Geometry: final body of the model. Coordinates: model frame, mm. A direction names the side the tool comes from. Round coordinates to 2 decimals unless told otherwise and drop trailing zeros. Loops run counter-clockwise (first coordinate to the right, second up) from the corner with the lowest first, then second, coordinate; pieces in that order, holes last. Notation, with made-up numbers: M 76,63.25 L 119,63.25 A18 cw 119,93.25 Z; hole C 67,16.25 d11. An arc over 180 degrees is marked long. Write each question's results on one line, items separated by ' | '.
```python
from build123d import *

# Parameters (mm, degrees)
F3_R     = 1.27
F4_DEPTH = 10.16
F6_R     = 15.24
F7_DEPTH = 2.54
F8_R     = 9.525
F8_R_2   = 2.6694227638
F9_DEPTH = 25.4


with BuildPart() as f1:
    # F0 (on Front) → F1 (revolve)
    with BuildSketch(Plane.XZ):
        with BuildLine():
            Line((0, 33.3398456074), (0, 38.1))
            ThreePointArc((0, 38.1), (-5.3715700607, 37.719441076), (-10.6358330914, 36.585366671))
            ThreePointArc((-10.6358330914, 36.585366671), (-5.5599989326, 34.1692827218), (0, 33.3398456074))
        make_face()
        with BuildLine():
            ThreePointArc((-10.6358330914, 36.585366671), (-5.3715700607, 37.719441076), (0, 38.1))
            Line((0, 38.1), (0, 67.6917069877))
            ThreePointArc((0, 67.6917069877), (-3.5141843979, 68.3636773923), (-6.5325309142, 70.2847761705))
            ThreePointArc((-6.5325309142, 70.2847761705), (-18.9103339688, 54.6924027056), (-10.6358330914, 36.585366671))
        make_face()
        with BuildLine():
            ThreePointArc((0, 33.3398456074), (-5.5599989326, 34.1692827218), (-10.6358330914, 36.585366671))
            ThreePointArc((-10.6358330914, 36.585366671), (-37.719441076, -5.3715700607), (0, -38.1))
            Line((0, -38.1), (0, 33.3398456074))
        make_face()
        with BuildLine():
            ThreePointArc((-6.5325309142, 70.2847761705), (-3.5141843979, 68.3636773923), (0, 67.6917069877))
            Line((0, 67.6917069877), (0, 71.4398456074))
            ThreePointArc((0, 71.4398456074), (-3.3169317731, 71.1488558055), (-6.5325309142, 70.2847761705))
        make_face()
        with BuildLine():
            ThreePointArc((0, 86.7417069877), (-8.8530295954, 80.7308913857), (-6.5325309142, 70.2847761705))
            ThreePointArc((-6.5325309142, 70.2847761705), (-3.3169317731, 71.1488558055), (0, 71.4398456074))
            Line((0, 71.4398456074), (0, 86.7417069877))
        make_face()
    revolve(axis=Axis((0, 0, 28.575), (0, 0, -1)))

    # F3 (on offset) → F4 (join)
    with BuildSketch(Plane.YZ):
        with BuildLine():
            ThreePointArc((1.27, 73.7371481955), (0.8980256121, 74.6351738076), (0, 75.0071481955))
            Line((0, 75.0071481955), (0, 72.4671481955))
            ThreePointArc((0, 72.4671481955), (0.8980256121, 72.8391225834), (1.27, 73.7371481955))
        make_face()
        with BuildLine():
            Line((0, 72.4671481955), (0, 75.0071481955))
            ThreePointArc((0, 75.0071481955), (-1.27, 73.7371481955), (0, 72.4671481955))
        make_face()
        with BuildLine():
            ThreePointArc((1.27, 78.1989917159), (0.8980256121, 79.097017328), (0, 79.4689917159))
            Line((0, 79.4689917159), (0, 76.9289917159))
            ThreePointArc((0, 76.9289917159), (0.8980256121, 77.3009661038), (1.27, 78.1989917159))
        make_face()
        with BuildLine():
            Line((0, 76.9289917159), (0, 79.4689917159))
            ThreePointArc((0, 79.4689917159), (-1.27, 78.1989917159), (0, 76.9289917159))
        make_face()
        with BuildLine():
            ThreePointArc((-5.3214693207, 82.12595433), (-3.4164693207, 80.22095433), (-1.5114693207, 82.12595433))
            Line((-1.5114693207, 82.12595433), (-5.3214693207, 82.12595433))
        make_face()
        with BuildLine():
            Line((-5.3214693207, 82.12595433), (-1.5114693207, 82.12595433))
            ThreePointArc((-1.5114693207, 82.12595433), (-3.4164693207, 84.03095433), (-5.3214693207, 82.12595433))
        make_face()
        with BuildLine():
            ThreePointArc((5.4735306793, 82.12595433), (3.5685306793, 84.03095433), (1.6635306793, 82.12595433))
            Line((1.6635306793, 82.12595433), (5.4735306793, 82.12595433))
        make_face()
        with BuildLine():
            Line((5.4735306793, 82.12595433), (1.6635306793, 82.12595433))
            ThreePointArc((1.6635306793, 82.12595433), (3.5685306793, 80.22095433), (5.4735306793, 82.12595433))
        make_face()
        with Locations((-7.385127712, 77.2191482013)):
            Circle(F3_R)
        with Locations((-4.0002781898, 74.8141407967)):
            Circle(F3_R)
        with Locations((7.0602684917, 77.3848402455)):
            Circle(F3_R)
        with Locations((3.981257522, 74.8031953548)):
            Circle(F3_R)
    extrude(amount=F4_DEPTH)

    # F6 (on offset) → F7 (join)
    with BuildSketch(Plane.XY.offset(83.82)):
        Circle(F6_R)
    extrude(amount=F7_DEPTH)

    # F8 (on face) → F9 (join)
    with BuildSketch(Plane.XY.offset(86.36)):
        Circle(F8_R)
        Circle(F8_R_2, mode=Mode.SUBTRACT)
    extrude(amount=F9_DEPTH)


solid = f1.part
```
1. Section B-B (y = -24). Output: boundary loops of the cut face in (x, z), then the cut area to 3 significant figures.
Answer key:
outline: C 0,0 d59.18 | area: 2,750 mm²
2. Pin query (flat end, axial travel): P1, Ø1.5, axis at x = 17.5, z = -13.5, coming from the +Y side; P2, Ø1.8, axis at y = -4, z = 82, coming from the +X side; P3, Ø3, axis at y = 3.5, z = 82.5, coming from the +X side. Return the tip coordinate at first contact, or that it passes through.
Answer key:
P1: stops at y = 31.55 | P2: stops at x = 10.16 | P3: stops at x = 14.98
3. Draft query along Y for faces 1 (the face through (10.16, -3, 82)), 2 (the face through (8.252, -5.265, 82.587)), 3 (the face through (-3.3, -14.88, 85.07)). Return one class per face: pulls with the +Y half, pulls with the -Y half, needs draft (parallel to the pull), parting line crosses it, or undercut.
Answer key:
face 1: needs draft | face 2: undercut | face 3: parting line crosses it
4. Section C-C (z = 2). Output: boundary loops of the cut face in (x, y).
Answer key:
outline: C 0,0 d76.09
5. Ray query, probe 1 along Y at (x, z) = (0, 92.5) (3 decimals); probe 2 along Y at (x, z) = (-1, 104); probe 3 along Z at (x, y) = (-22.5, -25). Return the intervals inside material, ascending.
Answer key:
probe 1: y = -9.525 to -2.669, 2.669 to 9.525 | probe 2: y = -9.47 to -2.48, 2.48 to 9.47 | probe 3: z = -17.9 to 17.9
6. Access query for faces 4 (the face through (-4, -7, 83.82)), 5 (the face through (2.546, 0.802, 98.882)), 6 (the face through (10.16, 4, 82)), 7 (the face through (2, -2, 111.76)). Directions: +Z, -Z, +X, -X, +Y, -Y. A direction counts if a zero-diameter tool reaches every point of the face in a straight line with its end or side. Return the directions, or none.
Answer key:
face 4: none | face 5: +Z | face 6: +X, +Y, -Y | face 7: +Z, +X, -X, +Y, -Y
7. Section A-A (x = 0). Output: boundary loops of the cut face in (y, z) (3 decimals).
Answer key:
outline: M -15.24,83.82 L -6.865,83.82 A9.525 ccw -6.533,70.285 A19.05 ccw -10.636,36.585 A38.1 ccw long 10.636,36.585 A19.05 ccw 6.533,70.285 A9.525 ccw 6.865,83.82 L 15.24,83.82 L 15.24,86.36 L 9.525,86.36 L 9.525,111.76 L 2.669,111.76 L 2.669,86.36 A9.525 ccw -2.669,86.36 L -2.669,111.76 L -9.525,111.76 L -9.525,86.36 L -15.24,86.36 Z
